Build history of the part. All positions in model axes, mm. Face numbers are marked on the shaded views. A direction names the side the tool comes from. Give positions to 0.01 mm unless a question says otherwise; leave off trailing zeros. Order: outer loops, then holes, each group sorted by start corner. A loop starts at its lowest first (then second) coordinate and runs counter-clockwise, first axis right, second up. Notation, with made-up numbers: (40.25, 10) - (55.25, 10) arc R8 cw to (55.25, 23) - close; hole circle Ø6 at (80, 5). An arc over 180 degrees is marked (long way). Use a Markdown table: item, result. Add a question column.
(1) Wall check: line 1 (Y direction, x = 84.7, z = 6); line 2 (Y direction, x = 54, z = 9.5); line 3 (X direction, y = 20, z = 21). Give the ranges that are in metal, low to high.
(2) Which spindle directions (+Z, -Z, +X, -X, +Y, -Y) get a long thin tool onto all of the face, cutting with end or side? Do the marked faces 1 and 2. Say none if no direction does.
(3) Slice it at A-A (z = 35). Write the cut outline in (x, y), then the cut area to 3 significant figures.
(4) Mould opens along X. For the marked faces 3, 4, 5 and 6 say: +X half, -X half, draft (parallel to the pull), parting line (faces both ways), or undercut.
(5) Flat gauge pins, fed straight in: pin 1 (2 mm diameter, centred on y = -14.5, z = 47.5, fed in from +X); pin 2 (1.5 mm diameter, centred on x = 15.5, z = 1.5, fed in from -Y); pin 3 (6 mm diameter, centred on y = -49, z = 6, fed in from +X). Where does each tip first touch, or does it go through?
(6) Slice it at B-B (y = 13). Write the cut outline in (x, z).
(7) Slice it at C-C (x = -4). Write the cut outline in (y, z).
(8) Slice it at D-D (y = -32.5). Write the cut outline in (x, z), then the cut area to 3 significant figures.
from build123d import *

# Parameters (mm, degrees)
BOSS_EXTRU_1_DEPTH       = 10
ENL_V_MAT_EXTRU_1_DEPTH  = 173.699160392
ESQUISSE6_W              = 170
ESQUISSE6_H              = 20.167534305
BOSS_EXTRU_2_DEPTH       = 2
ESQUISSE8_W              = 185.001498893
ESQUISSE8_H              = 2
BOSS_EXTRU_3_DEPTH       = 50
ESQUISSE9_W              = 70
ESQUISSE9_H              = 152
BOSS_EXTRU_4_DEPTH       = 2
ESQUISSE10_W             = 69.947510153
ESQUISSE10_H             = 152
BOSS_EXTRU_5_DEPTH       = 2
ESQUISSE11_W             = 58
ESQUISSE11_H             = 20
BOSS_EXTRU_6_DEPTH       = 2
ESQUISSE19_W             = 64
ESQUISSE19_H             = 70.167534305
ENL_V_MAT_EXTRU_9_DEPTH  = 2
ESQUISSE24_R             = 2.5
ENL_V_MAT_EXTRU_10_DEPTH = 3
ENL_V_MAT_EXTRU_11_DEPTH = 3
ESQUISSE27_W             = 13.001498893
ESQUISSE27_H             = 50.044295801
ENL_V_MAT_EXTRU_12_DEPTH = 196.007134873
ESQUISSE28_W             = 70.169211379
ESQUISSE28_H             = 154
ENL_V_MAT_EXTRU_13_DEPTH = 2
ESQUISSE29_W             = 10
ESQUISSE29_H             = 90
BOSS_EXTRU_7_DEPTH       = 2
ESQUISSE30_W             = 1.763859519
ESQUISSE30_H             = 90
BOSS_EXTRU_8_DEPTH       = 10


with BuildPart() as part:
    # Esquisse1 → Boss.-Extru.1 (new body)
    with BuildSketch(Plane.XY):
        Polygon((-29, 27), (-29, 75), (-85, 75), (-85, -75), (85, -75), (85, 75), (29, 75), (29, 27), align=None)
    extrude(amount=BOSS_EXTRU_1_DEPTH)

    # Esquisse5 → Enlèv. mat.-Extru.1 (cut, through all)
    with BuildSketch(Plane.XZ.offset(75)):
        Polygon((-85, 10), (85, 10), (0, 2), align=None)
    extrude(amount=-ENL_V_MAT_EXTRU_1_DEPTH, mode=Mode.SUBTRACT)

    # Esquisse6 → Boss.-Extru.2 (add)
    with BuildSketch(Plane(origin=(0, -75, 0), x_dir=(-1, 0, 0), z_dir=(0, -1, 0))):
        with Locations((0, -10.083767153)):
            Rectangle(ESQUISSE6_W, ESQUISSE6_H)
    extrude(amount=BOSS_EXTRU_2_DEPTH)

    # Esquisse8 → Boss.-Extru.3 (add)
    with BuildSketch(Plane.XY.offset(20.167534305)):
        with Locations((7.500749447, -76)):
            Rectangle(ESQUISSE8_W, ESQUISSE8_H)
    extrude(amount=BOSS_EXTRU_3_DEPTH)

    # Esquisse9 → Boss.-Extru.4 (add)
    with BuildSketch(Plane.ZY.offset(85)):
        with Locations((35, -1)):
            Rectangle(ESQUISSE9_W, ESQUISSE9_H)
    extrude(amount=BOSS_EXTRU_4_DEPTH)

    # Esquisse10 → Boss.-Extru.5 (add)
    with BuildSketch(Plane(origin=(85, 0, 0), x_dir=(0, 0, -1), z_dir=(1, 0, 0))):
        with Locations((-34.973755077, -1)):
            Rectangle(ESQUISSE10_W, ESQUISSE10_H)
    extrude(amount=BOSS_EXTRU_5_DEPTH)

    # Esquisse11 → Boss.-Extru.6 (add)
    with BuildSketch(Plane(origin=(0, 75, 0), x_dir=(1, 0, 0), z_dir=(0, 1, 0))):
        with Locations((-58, -10)):
            Rectangle(ESQUISSE11_W, ESQUISSE11_H)
        with Locations((58, -10)):
            Rectangle(ESQUISSE11_W, ESQUISSE11_H)
    extrude(amount=BOSS_EXTRU_6_DEPTH)

    # Esquisse19 → Enlèv. mat.-Extru.9 (cut)
    with BuildSketch(Plane(origin=(0, -77, 0), x_dir=(-1, 0, 0), z_dir=(0, -1, 0))):
        with Locations((0, -35.083767153)):
            Rectangle(ESQUISSE19_W, ESQUISSE19_H)
    extrude(amount=-ENL_V_MAT_EXTRU_9_DEPTH, mode=Mode.SUBTRACT)

    # Esquisse24 → Enlèv. mat.-Extru.10 (cut)
    with BuildSketch(Plane(origin=(87, 0, 0), x_dir=(0, 0, -1), z_dir=(1, 0, 0))):
        with Locations((-6, -49)):
            Circle(ESQUISSE24_R)
    extrude(amount=-ENL_V_MAT_EXTRU_10_DEPTH, mode=Mode.SUBTRACT)

    # Esquisse25 → Enlèv. mat.-Extru.11 (cut)
    with BuildSketch(Plane.ZY.offset(87)):
        Polygon((6, -51.886751346), (8.5, -50.443375673), (8.5, -47.556624327), (6, -46.113248654), (3.5, -47.556624327), (3.5, -50.443375673), align=None)
    extrude(amount=-ENL_V_MAT_EXTRU_11_DEPTH, mode=Mode.SUBTRACT)

    # Esquisse27 → Enlèv. mat.-Extru.12 (cut, through all)
    with BuildSketch(Plane(origin=(0, -75, 0), x_dir=(1, 0, 0), z_dir=(0, 1, 0))):
        with Locations((93.500749447, -45.189682206)):
            Rectangle(ESQUISSE27_W, ESQUISSE27_H)
    extrude(amount=-ENL_V_MAT_EXTRU_12_DEPTH, mode=Mode.SUBTRACT)

    # Esquisse28 → Enlèv. mat.-Extru.13 (cut)
    with BuildSketch(Plane(origin=(87, 0, 0), x_dir=(0, 0, -1), z_dir=(1, 0, 0))):
        with Locations((-35.08460569, 0)):
            Rectangle(ESQUISSE28_W, ESQUISSE28_H)
    extrude(amount=-ENL_V_MAT_EXTRU_13_DEPTH, mode=Mode.SUBTRACT)

    # Esquisse29 → Boss.-Extru.7 (add)
    with BuildSketch(Plane(origin=(85, 0, 0), x_dir=(0, 0, -1), z_dir=(1, 0, 0))):
        with Locations((-5, 32.051779958)):
            Rectangle(ESQUISSE29_W, ESQUISSE29_H)
    extrude(amount=BOSS_EXTRU_7_DEPTH)

    # Esquisse30 → Boss.-Extru.8 (add)
    with BuildSketch(Plane.XY.offset(10)):
        with Locations((86.118070241, 32.051779958)):
            Rectangle(ESQUISSE30_W, ESQUISSE30_H)
    extrude(amount=BOSS_EXTRU_8_DEPTH)


solid = part.part
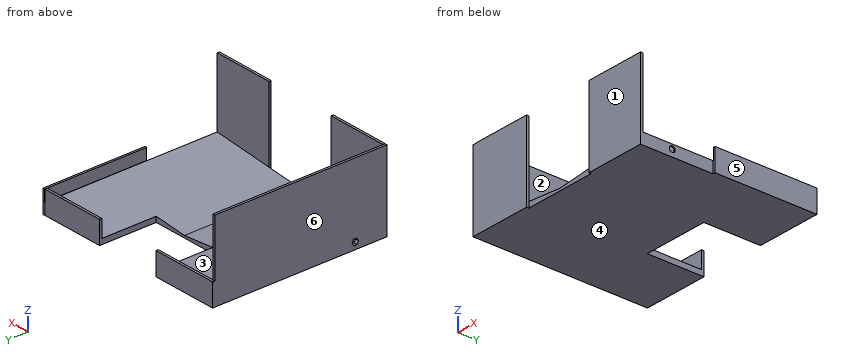
Solution:
| question | item | result |
|---|---|---|
| 1 | line 1 | -77 to -51.5, -46.5 to 77 |
| 1 | line 2 | -77 to -75, 75 to 77 |
| 1 | line 3 | -87 to -85 |
| 2 | face 1 | +Z, -Z, +X, -X, -Y |
| 2 | face 2 | +Z |
| 3 | outline | (-87, -77) - (-32, -77) - (-32, -75) - (-85, -75) - (-85, 75) - (-87, 75) - close; (32, -77) - (85, -77) - (85, -75) - (32, -75) - close |
| 3 | area | 516 mm2 |
| 4 | face 3 | undercut |
| 4 | face 4 | draft |
| 4 | face 5 | +X half |
| 4 | face 6 | -X half |
| 5 | pin 1 | x = -85 |
| 5 | pin 2 | y = -75 |
| 5 | pin 3 | x = 85 |
| 6 | outline | (-87, 0) - (87, 0) - (87, 20) - (85.24, 20) - (85.24, 10) - (85, 10) - (0, 2) - (-85, 10) - (-85, 70) - (-87, 70) - close |
| 7 | outline | (-75, 0) - (27, 0) - (27, 2.38) - (-75, 2.38) - close |
| 8 | outline | (-87, 0) - (85, 0) - (85, 10) - (0, 2) - (-85, 10) - (-85, 70) - (-87, 70) - close |
| 8 | area | 1,160 mm2 |
